Drawing for the job (mm, zero at the part's lowest x, y, z). Give positions to 0.01 mm unless a question says otherwise; leave off trailing zeros. Order: outer loops, then holes, each group sorted by start corner. A loop starts at its lowest first (then second) coordinate and runs counter-clockwise, first axis right, second up. Notation, with made-up numbers: (64.5, -30) - (95.5, -30) arc R17 ccw to (95.5, -21) - close; hole circle Ø5 at (84.5, 7). An arc over 180 degrees is marked (long way). Use a Markdown table: item, result.
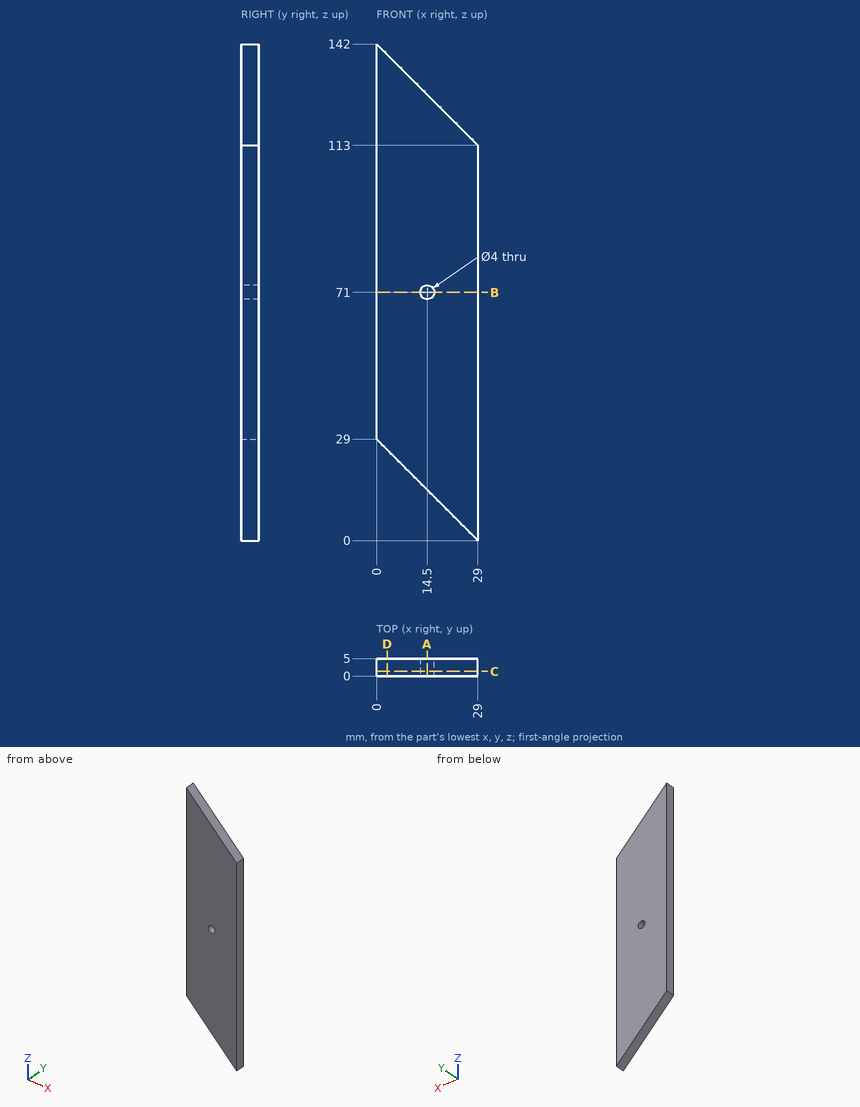
1) Slice it at B-B (z = 71). Write the cut outline in (x, y).
Computed:
| item | result |
|---|---|
| outline | (0, 0) - (12.5, 0) - (12.5, 5) - (0, 5) - close; (16.5, 0) - (29, 0) - (29, 5) - (16.5, 5) - close |
2) Slice it at A-A (x = 14.5). Write the cut outline in (y, z).
Computed:
| item | result |
|---|---|
| outline | (0, 14.5) - (5, 14.5) - (5, 69) - (0, 69) - close; (0, 73) - (5, 73) - (5, 127.5) - (0, 127.5) - close |
3) Slice it at C-C (y = 1.3). Write the cut outline in (x, z), and give its area (3 significant figures).
Computed:
| item | result |
|---|---|
| outline | (0, 29) - (29, 0) - (29, 113) - (0, 142) - close; hole circle Ø4 at (14.5, 71) |
| area | 3,260 mm² |
4) Pin check, flat tips, straight feed: P1, Ø5, axis at x = 14.5, z = 71, coming from the -Y side; P2, Ø1, axis at x = 25, y = 2, coming from the -Z side; P3, Ø1, axis at x = 22, y = 3, coming from the +Z side. Stop position of each tip, or through.
Computed:
| item | result |
|---|---|
| P1 | stops at y = 0 |
| P2 | stops at z = 3.5 |
| P3 | stops at z = 120.5 |
5) Wall check: line 1 (X direction, y = 3.75, z = 71); line 2 (Z direction, x = 14.5, y = 3); line 3 (Z direction, x = 17, y = 1.9). Give the ranges that are in metal, low to high. Write a range as from..to.
Computed:
| item | result |
|---|---|
| line 1 | x = 0..12.5, 16.5..29 |
| line 2 | z = 14.5..69, 73..127.5 |
| line 3 | z = 12..125 |
6) Slice it at D-D (x = 3). Write the cut outline in (y, z), and give its area (3 significant figures).
Computed:
| item | result |
|---|---|
| outline | (0, 26) - (5, 26) - (5, 139) - (0, 139) - close |
| area | 565 mm² |
